from build123d import *

# Parameters (mm, degrees)
F0_W     = 43.873566
F0_H     = 39.735638
F1_DEPTH = 67.251692
F2_SIZE  = 5.08
F3_R     = 4.729386
F4_DEPTH = 50.0404


with BuildPart() as f1:
    # F0 (on Top) → F1 (new body)
    with BuildSketch(Plane.XY):
        with Locations((4.820467, -19.867819)):
            Rectangle(F0_W, F0_H)
    extrude(amount=F1_DEPTH)

    # F2
    f2_edges = [f1.edges().sort_by_distance(p)[0] for p in [
        (26.75725, -39.735638, 33.625846),
        (26.75725, -19.867819, 67.251692),
        (4.820467, -39.735638, 67.251692),
        (-17.116316, -19.867819, 67.251692),
        (-17.116316, -39.735638, 33.625846),
        (-17.116316, -19.867819, 0),
        (26.75725, -19.867819, 0),
        (4.820467, 0, 0),
        (26.75725, 0, 33.625846),
        (-17.116316, 0, 33.625846),
        (4.820467, 0, 67.251692),
        (4.820467, -39.735638, 0),
    ]]
    chamfer(f2_edges, length=F2_SIZE)

    # F3 (on face) → F4 (join)
    with BuildSketch(Plane.XY.offset(67.251692)):
        with Locations((0, -16.326718)):
            Circle(F3_R)
    extrude(amount=F4_DEPTH)


solid = f1.part
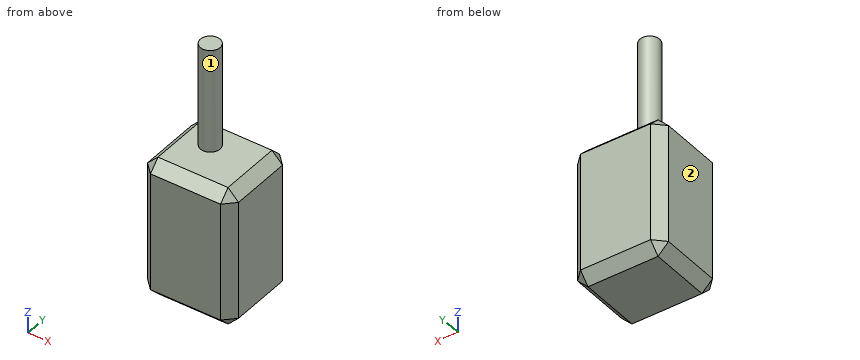
Model file for the job. Use its own axes, mm. Face numbers are marked on the shaded views. A direction names the side the tool comes from. Coordinates: 2 decimals unless noted, no trailing zeros. Order: outer loops, then holes, each group sorted by start corner. A loop starts at its lowest first (then second) coordinate and runs counter-clockwise, first axis right, second up. Notation, with made-up numbers: (84.25, 43.5) -> (115.25, 43.5) arc R13 ccw to (115.25, 57.5) -> close; hole circle Ø10 at (-22.75, 64.5). An arc over 180 degrees is marked (long way). Return JSON: item names as keys, results as strings. Group by question number.
Item 1: Saw through at D-D on z = 88.5. Write the cut outline in (x, y), then the cut area to 3 significant figures.
Item 2: Tool access for the marked faces 1 and 2: list every direction of +Z, -Z, +X, -X, +Y, -Y with a clear straight run to the whole face (end or side of a thin tool).
Item 3: Saw through at A-A on y = -7. Write the cut outline in (x, z), then the cut area to 3 significant figures.
Item 4: Saw through at B-B on z = 15. Write the cut outline in (x, y), then the cut area to 3 significant figures.
Item 5: Wall check: line 1 along Z through (x, y) = (20.5, -32); line 2 along Z through (x, y) = (-15, -36.5); line 3 along Y through (x, z) = (3.5, 79.5). Give the ranges that are in metal, low to high. Write a range as [from, to].
Item 6: Flat gauge pins, fed straight in: P1, Ø4, axis at x = 8, z = 71, coming from the -Y side; P2, Ø3, axis at x = -12.5, y = -20.5, coming from the +Z side; P3, Ø6, axis at x = 5, z = 98, coming from the -Y side. Where does each tip first touch, or does it go through?
Item 7: Saw through at C-C on x = 0. Write the cut outline in (y, z), then the cut area to 3 significant figures.
Values found:
{
 "1": {"outline": "circle Ø9.46 at (0, -16.33)", "area": "70.3 mm2"},
 "2": {"face 1": "+Z", "face 2": "+Z, -Z, -X, +Y, -Y"},
 "3": {"outline": "(-17.12, 5.08) -> (-12.04, 0) -> (21.68, 0) -> (26.76, 5.08) -> (26.76, 62.17) -> (21.68, 67.25) -> (-12.04, 67.25) -> (-17.12, 62.17) -> close", "area": "2,900 mm2"},
 "4": {"outline": "(-17.12, -34.66) -> (-12.04, -39.74) -> (21.68, -39.74) -> (26.76, -34.66) -> (26.76, -5.08) -> (21.68, 0) -> (-12.04, 0) -> (-17.12, -5.08) -> close", "area": "1,690 mm2"},
 "5": {"line 1": "z = [0, 67.25]", "line 2": "z = [4.81, 62.44]", "line 3": "y = [-19.51, -13.15]"},
 "6": {"P1": "passes through", "P2": "stops at z = 67.25", "P3": "stops at y = -20.61"},
 "7": {"outline": "(-39.74, 5.08) -> (-34.66, 0) -> (-5.08, 0) -> (0, 5.08) -> (0, 62.17) -> (-5.08, 67.25) -> (-11.6, 67.25) -> (-11.6, 117.29) -> (-21.06, 117.29) -> (-21.06, 67.25) -> (-34.66, 67.25) -> (-39.74, 62.17) -> close", "area": "3,090 mm2"}
}
